The model under review builds one solid part; all positions refer to its coordinate system, in mm. A direction names the side the tool comes from. Round coordinates to 2 decimals unless told otherwise and drop trailing zeros. Order: outer loops, then holes, each group sorted by start corner. A loop starts at its lowest first (then second) coordinate and runs counter-clockwise, first axis right, second up. Notation, with made-up numbers: M 68.5,16.5 L 87.5,16.5 A17 ccw 87.5,25.5 Z; hole C 76.5,76 d2. An arc over 180 degrees is marked long. Use a Markdown table: item, result. Add a question column.
1. The part is to be moulded in two halves that separate along X. For faces 4 (the cylindrical face through (39.95, 27.41, 0.74)), 5 (the flat face through (68.8, -1, 1)), 6 (the flat face through (41, 0, 0)), say which applies: +X half, -X half, draft (parallel to the pull), parting line (faces both ways), or undercut.
2. Consider section A-A on x = 41.3. State the section outline as (y, z) points.
3. For faces 1 (the flat face through (36.3, -30, 1)), 2 (the flat face through (58, -26.15, 1)), 3 (the flat face through (36.3, 29, 1)), list the 3-axis set-ups (+Z, -Z, +X, -X, +Y, -Y) from which the entire face can be reached by the end or side of a thin tool; tool diameter is ignored.
4. To check wall thickness, follow probe 1 along Y at (x, z) = (41.3, 0.7); probe 2 along Y at (x, z) = (42, 0.35); probe 3 along Y at (x, z) = (22, 1.8). State the ranges of each line that lie inside material, in increasing order.
5. Insertion check: P1, Ø12, axis at x = 62, y = -19.5, coming from the -Z side; P2, Ø2.5, axis at x = 41.3, y = -27.65, coming from the -Z side; P3, Ø1.5, axis at x = 26.5, z = 1.5, coming from the -Y side; P4, Ø0.9, axis at y = 29.5, z = 1, coming from the +X side. Each pin has a flat end and moves straight along its axis. Give the tip position at first contact, or say it passes through.
6. Consider section C-C on x = 55. State the section outline as (y, z) points, then the cut area to 3 significant figures.
7. Consider section B-B on z = 0.45. State the section outline as (x, y) points.
from build123d import *

# Parameters (mm, degrees)
SKETCH_1_R      = 1.35
EXTRUDE_1_DEPTH = 3
CHAMFER_1_SIZE  = 1.5


with BuildPart() as part:
    # Эскиз1 → Бобышка-Вытянуть1 (new body)
    with BuildSketch(Plane.XY):
        with BuildLine():
            Line((68.8, 25.85), (48.3, 25.85))
            ThreePointArc((48.3, 25.85), (46.885786438, 26.435786438), (46.3, 27.85))
            Line((46.3, 27.85), (46.3, 30.84491535))
            Line((46.3, 30.84491535), (36.3, 30.84491535))
            Line((36.3, 30.84491535), (36.3, 27.85))
            ThreePointArc((36.3, 27.85), (35.714213562, 26.435786438), (34.3, 25.85))
            Line((34.3, 25.85), (13.8, 25.85))
            Line((13.8, 25.85), (13.8, -26.15))
            Line((13.8, -26.15), (34.3, -26.15))
            ThreePointArc((34.3, -26.15), (35.714213562, -26.735786438), (36.3, -28.15))
            Line((36.3, -28.15), (36.3, -31.15))
            Line((36.3, -31.15), (46.3, -31.15))
            Line((46.3, -31.15), (46.3, -28.15))
            ThreePointArc((46.3, -28.15), (46.885786438, -26.735786438), (48.3, -26.15))
            Line((48.3, -26.15), (68.8, -26.15))
            Line((68.8, -26.15), (68.8, 25.85))
        make_face()
        with Locations((41.3, 27.347457675)):
            Circle(SKETCH_1_R, mode=Mode.SUBTRACT)
        with Locations((41.3, -27.652542325)):
            Circle(SKETCH_1_R, mode=Mode.SUBTRACT)
    extrude(amount=EXTRUDE_1_DEPTH)

    # Фаска1
    chamfer_1_edges = [part.edges().sort_by_distance(p)[0] for p in [
        (39.95, -27.652542325, 3),
        (39.95, 27.347457675, 3),
    ]]
    chamfer(chamfer_1_edges, length=CHAMFER_1_SIZE)


solid = part.part
Answer block:
| question | item | result |
|---|---|---|
| 1 | face 4 | undercut |
| 1 | face 5 | +X half |
| 1 | face 6 | draft |
| 2 | outline | M -31.15,0 L -29,0 L -29,1.5 L -30.5,3 L -31.15,3 Z; M -26.3,0 L 26,0 L 26,1.5 L 24.5,3 L -24.8,3 L -26.3,1.5 Z; M 28.7,0 L 30.84,0 L 30.84,3 L 30.2,3 L 28.7,1.5 Z |
| 3 | face 1 | +Z, -Z, -X, -Y |
| 3 | face 2 | +Z, -Z, +X, -Y |
| 3 | face 3 | +Z, -Z, -X, +Y |
| 4 | probe 1 | -31.15 to -29, -26.3 to 26, 28.7 to 30.84 |
| 4 | probe 2 | -31.15 to -28.81, -26.5 to 26.19, 28.5 to 30.84 |
| 4 | probe 3 | -26.15 to 25.85 |
| 5 | P1 | z = 0 |
| 5 | P2 | through |
| 5 | P3 | y = -26.15 |
| 5 | P4 | x = 46.3 |
| 6 | outline | M -26.15,0 L 25.85,0 L 25.85,3 L -26.15,3 Z |
| 6 | area | 156 mm^2 |
| 7 | outline | M 13.8,-26.15 L 34.3,-26.15 A2 cw 36.3,-28.15 L 36.3,-31.15 L 46.3,-31.15 L 46.3,-28.15 A2 cw 48.3,-26.15 L 68.8,-26.15 L 68.8,25.85 L 48.3,25.85 A2 cw 46.3,27.85 L 46.3,30.84 L 36.3,30.84 L 36.3,27.85 A2 cw 34.3,25.85 L 13.8,25.85 Z; hole C 41.3,-27.65 d2.7; hole C 41.3,27.35 d2.7 |
